```python
from build123d import *

# Parameters (mm, degrees)
PAD010_DEPTH    = 9
FILLET029_R     = 6.5
FILLET030_R     = 4
FILLET031_R     = 1
FILLET032_R     = 1
FILLET033_R     = 2
FILLET034_R     = 4
SKETCH043_R     = 1.7
POCKET021_DEPTH = 9
FILLET040_R     = 6
FILLET041_R     = 32
FILLET042_R     = 1


with BuildPart() as part:
    # Sketch040 → Pad010 (new body)
    with BuildSketch(Plane.XZ):
        Polygon((-18.1, 39.4), (-18.1, 21.0678404338), (-11.6, 21.0678404338), (-11.6, 32.9), (-0.4644712743, 32.9), (-0.4644712743, 28.9), (2.5355287257, 28.9), (5.0833203655, 35.9), (19, 35.9), (19, 31.2), (17, 31.2), (17, 28.4), (19, 26.4), (23.5, 26.4), (23.5, 32.9), (33.481928, 39.806227), (33.5, 42.499247), (23.5, 39.4), align=None)
    extrude(amount=-PAD010_DEPTH)

    # Fillet029
    fillet029_edges = [part.edges().sort_by_distance(p)[0] for p in [
        (-18.1, 4.5, 39.4),
    ]]
    fillet(fillet029_edges, radius=FILLET029_R)

    # Fillet030
    fillet030_edges = [part.edges().sort_by_distance(p)[0] for p in [
        (-11.6, 4.5, 21.06784),
    ]]
    fillet(fillet030_edges, radius=FILLET030_R)

    # Fillet031
    fillet031_edges = [part.edges().sort_by_distance(p)[0] for p in [
        (-0.464471, 4.5, 28.9),
    ]]
    fillet(fillet031_edges, radius=FILLET031_R)

    # Fillet032
    fillet032_edges = [part.edges().sort_by_distance(p)[0] for p in [
        (-0.464471, 4.5, 32.9),
        (19, 4.5, 35.9),
        (2.535529, 4.5, 28.9),
        (23.5, 4.5, 26.4),
        (19, 4.5, 26.4),
        (-18.1, 4.5, 21.06784),
        (19, 4.5, 31.2),
    ]]
    fillet(fillet032_edges, radius=FILLET032_R)

    # Fillet033
    fillet033_edges = [part.edges().sort_by_distance(p)[0] for p in [
        (5.08332, 4.5, 35.9),
    ]]
    fillet(fillet033_edges, radius=FILLET033_R)

    # Fillet034
    fillet034_edges = [part.edges().sort_by_distance(p)[0] for p in [
        (17, 4.5, 28.4),
    ]]
    fillet(fillet034_edges, radius=FILLET034_R)

    # Sketch043 (on Face1 of Fillet033) → Pocket021 (cut)
    with BuildSketch(Plane.XZ):
        with Locations((-11.6, 32.9)):
            Circle(SKETCH043_R)
    extrude(amount=-POCKET021_DEPTH, mode=Mode.SUBTRACT)

    # Fillet040
    fillet040_edges = [part.edges().sort_by_distance(p)[0] for p in [
        (23.5, 4.5, 32.9),
    ]]
    fillet(fillet040_edges, radius=FILLET040_R)

    # Fillet041
    fillet041_edges = [part.edges().sort_by_distance(p)[0] for p in [
        (23.5, 4.5, 39.4),
    ]]
    fillet(fillet041_edges, radius=FILLET041_R)

    # Fillet042
    fillet042_edges = [part.edges().sort_by_distance(p)[0] for p in [
        (33.481928, 4.5, 39.806227),
        (33.5, 4.5, 42.499247),
    ]]
    fillet(fillet042_edges, radius=FILLET042_R)


with BuildPart() as part_1:
    # Body008 placement: moved
    add(part.part.moved(Location((-0.4, 0, 0.1))))


solid = part_1.part
```
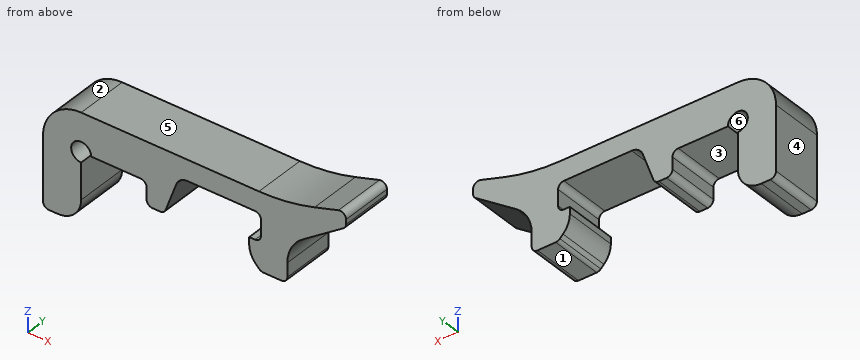
Verification items for the finished model (mm, model axes). Face numbers are marked on the shaded views. A direction names the side the tool comes from. Give positions to 0.01 mm unless a question says otherwise; leave off trailing zeros. Order: outer loops, then holes, each group sorted by start corner. A loop starts at its lowest first (then second) coordinate and runs counter-clockwise, first axis right, second up. Notation, with made-up numbers: M 44.5,76 L 62.5,76 A22 cw 62.5,91 Z; hole C 30,81 d8. An arc over 180 degrees is marked long. Answer in a Markdown table with one row per item. Add a question column.
Item 1: Section check A-A, the plane z = 28.5. Enter the section's corners in (x, y), and give its area (3 significant figures).
Item 2: Gauge pin test, flat ends, axial feed: pin 1 (0.7 mm diameter, centred on y = 4, z = 29, fed in from +X); pin 2 (2 mm diameter, centred on y = 3, z = 40, fed in from -X); pin 3 (5 mm diameter, centred on y = 5.5, z = 29.5, fed in from +X). Record the tip position at first contact, or that the pin passes through.
Item 3: Scan lines: probe 1 along X at (y, z) = (1.75, 25.25); probe 2 along X at (y, z) = (2.25, 35); probe 3 along X at (y, z) = (8, 27). Record each from-to range of solid material in increasing order. Write a range as from..to.
Item 4: Tool access check on the marked faces 1, 2 and 3. Record the directions out of +Z, -Z, +X, -X, +Y, -Y that give a thin tool (end or side, any length) a straight path to the whole face; none if there is none.
Item 5: Mould release check, pull along Z, two halves, no side actions. Record for the marked faces 4, 5 and 6: released by +Z, released by -Z, zero draft, split by the parting line, or undercut.
Item 6: Section check B-B, the plane x = 11.5. Enter the section's corners in (y, z).
Item 7: Section check C-C, the plane x = -8. Enter the section's corners in (y, z), and give its area (3 significant figures).
Filled sheet:
| question | item | result |
|---|---|---|
| 1 | outline | M -18.5,0 L -12,0 L -12,9 L -18.5,9 Z; M 16.96,0 L 23.1,0 L 23.1,9 L 16.96,9 Z |
| 1 | area | 114 mm^2 |
| 2 | pin 1 | stops at x = 23.1 |
| 2 | pin 2 | stops at x = -14.5 |
| 2 | pin 3 | stops at x = 23.5 |
| 3 | probe 1 | x = -18.5..-12 |
| 3 | probe 2 | x = -18.18..4.35, 18.6..25.99 |
| 3 | probe 3 | x = -18.5..-12, 18.1..22.97 |
| 4 | face 1 | -Z, +X, +Y, -Y |
| 4 | face 2 | +Z, -X, +Y, -Y |
| 4 | face 3 | -Z, +Y, -Y |
| 5 | face 4 | zero draft |
| 5 | face 5 | released by +Z |
| 5 | face 6 | undercut |
| 6 | outline | M 0,36 L 9,36 L 9,39.5 L 0,39.5 Z |
| 7 | outline | M 0,33 L 9,33 L 9,39.5 L 0,39.5 Z |
| 7 | area | 58.5 mm^2 |
